from build123d import *

# Parameters (mm, degrees)
SKETCH1_W                       = 96.52
SKETCH1_H                       = 39.878
BOSS_EXTRUDE1_DEPTH             = 3
F_32_0_116_DIAMETER_HOLE1_D     = 2.9464
F_32_0_116_DIAMETER_HOLE1_DEPTH = 1.524
F_32_0_116_DIAMETER_HOLE1_TIP   = 0.885187864
CUT_EXTRUDE1_DEPTH              = 3
FILLET1_R                       = 2.54
SKETCH5_W                       = 12.7
SKETCH5_H                       = 3
CUT_EXTRUDE2_DEPTH              = 3


with BuildPart() as part:
    # Sketch1 → Boss-Extrude1 (new body)
    with BuildSketch(Plane(origin=(0, 0, 0), x_dir=(0, 0, -1), z_dir=(1, 0, 0))):
        with Locations((48.26, 19.939)):
            Rectangle(SKETCH1_W, SKETCH1_H)
    extrude(amount=BOSS_EXTRUDE1_DEPTH)

    # #32 (0.116) Diameter Hole1
    with Locations(Plane(origin=(3, 0, 0), x_dir=(0, 0, -1), z_dir=(1, 0, 0))):
        with Locations((48.26, 6.35)):
            Hole(F_32_0_116_DIAMETER_HOLE1_D / 2, depth=F_32_0_116_DIAMETER_HOLE1_DEPTH)
            with Locations((0, 0, -(F_32_0_116_DIAMETER_HOLE1_DEPTH + F_32_0_116_DIAMETER_HOLE1_TIP / 2))):  # 118° drill point
                Cone(0, F_32_0_116_DIAMETER_HOLE1_D / 2, F_32_0_116_DIAMETER_HOLE1_TIP, mode=Mode.SUBTRACT)

    # Sketch4 → Cut-Extrude1 (cut)
    with BuildSketch(Plane(origin=(3, 0, 0), x_dir=(0, 0, -1), z_dir=(1, 0, 0))):
        Polygon((0, 34.338), (5.08, 34.338), (5.08, 35.88105), (7.46125, 35.88105), (7.46125, 34.338), (10.16, 34.338), (10.16, 31.0741), (7.46125, 31.0741), (7.46125, 29.53105), (5.08, 29.53105), (5.08, 31.0741), (0, 31.0741), align=None)
        Polygon((96.52, 31.0741), (96.52, 34.338), (91.44, 34.338), (91.44, 35.88105), (89.05875, 35.88105), (89.05875, 34.338), (86.36, 34.338), (86.36, 31.0741), (89.05875, 31.0741), (89.05875, 29.53105), (91.44, 29.53105), (91.44, 31.0741), align=None)
    extrude(amount=-CUT_EXTRUDE1_DEPTH, mode=Mode.SUBTRACT)

    # Fillet1
    fillet1_edges = [part.edges().sort_by_distance(p)[0] for p in [
        (1.5, 0, -96.52),
        (1.5, 0, 0),
    ]]
    fillet(fillet1_edges, radius=FILLET1_R)

    # Sketch5 → Cut-Extrude2 (cut)
    with BuildSketch(Plane(origin=(3, 0, 0), x_dir=(0, 0, -1), z_dir=(1, 0, 0))):
        with Locations((48.26, 38.378)):
            Rectangle(SKETCH5_W, SKETCH5_H)
    extrude(amount=-CUT_EXTRUDE2_DEPTH, mode=Mode.SUBTRACT)


solid = part.part
Could you check a few things on this model? Use its own coordinates, in mm. A direction names the side the tool comes from. Give positions to 0.01 mm unless a question says otherwise; leave off trailing zeros. Order: outer loops, then holes, each group sorted by start corner. A loop starts at its lowest first (then second) coordinate and runs counter-clockwise, first axis right, second up.
1. Will this pin go through, and if not, where does the flat tip stop? P1, Ø2.5, axis at y = 6.35, z = -48.26, coming from the +X side.
2. We'd pull the mould along Z, two halves only. Please class faces 4 (the flat face through (2, 29.531, -6)), 5 (the flat face through (2, 31.074, -9)), 6 (the flat face through (1, 37, 0)): pulls with the +Z half, pulls with the -Z half, needs draft (parallel to the pull), parting line crosses it, or undercut.
3. I need wall thicknesses on L1, parallel to Y at x = 0.3, z = -8.5; L2, parallel to Y at x = 2.25, z = -48.26; L3, parallel to Z at x = 2.65, y = 6.35. Which ranges of each line are inside material? Lowest first, please.
4. Suppose I cut it at A-A (y = 32.5). List the corners of the cut face in (x, z) for me, plus the area to 3 significant figures.
5. Suppose I cut it at B-B (z = -52.5). List the corners of the cut face in (x, y) for me, plus the area to 3 significant figures.
6. For faces 1 (the flat face through (2, 38, -41.91)), 2 (the flat face through (2, 35.881, -90)), 3 (the flat face through (2, 34.338, -94)), which set-ups out of +Z, -Z, +X, -X, +Y, -Y let a thin tool reach every point of the face, with its end or its side?
Solved:
1. P1: stops at x = 1.34
2. face 4: undercut
2. face 5: needs draft
2. face 6: pulls with the +Z half
3. L1: y = 0 to 31.07, 34.34 to 39.88
3. L2: y = 0 to 4.88, 7.82 to 36.88
3. L3: z = -96.52 to -49.73, -46.79 to 0
4. outline: (0, -86.36) - (3, -86.36) - (3, -10.16) - (0, -10.16) - close
4. area: 229 mm2
5. outline: (0, 0) - (3, 0) - (3, 36.88) - (0, 36.88) - close
5. area: 111 mm2
6. face 1: +X, -X, +Y
6. face 2: +X, -X
6. face 3: -Z, +X, -X
